Geometry check sheet. Reference: the model listing, model coordinates, mm. A direction names the side the tool comes from. Round coordinates to 2 decimals unless told otherwise and drop trailing zeros. Loops run counter-clockwise (first coordinate to the right, second up) from the corner with the lowest first, then second, coordinate; pieces in that order, holes last. Notation, with made-up numbers: (0, -33) - (59, -33) arc R25 ccw to (59, 2) - close; hole circle Ø10 at (-2, -14.5). An arc over 180 degrees is marked (long way). Write item = value, one per line.
```python
from build123d import *

# Parameters (mm, degrees)
SKETCH_W        = 22
SKETCH_H        = 30
PAD_DEPTH       = 27
SKETCH001_W     = 22
SKETCH001_H     = 28
PAD001_DEPTH    = 30
PAD002_DEPTH    = 4
SKETCH003_R     = 5
PAD003_DEPTH    = 4
PAD004_DEPTH    = 17
SKETCH005_R     = 7
PAD005_DEPTH    = 3
SKETCH006_R     = 4
POCKET_DEPTH    = 30
SKETCH007_W     = 15
SKETCH007_H     = 6
PAD006_DEPTH    = 5
SKETCH008_R     = 5
PAD007_DEPTH    = 4
PAD008_DEPTH    = 17
SKETCH010_R     = 7
PAD009_DEPTH    = 3
SKETCH011_R     = 4
POCKET001_DEPTH = 30
SKETCH012_R     = 2
POCKET002_DEPTH = 5


with BuildPart() as part:
    # Sketch → Pad (new body)
    with BuildSketch(Plane.XY):
        Rectangle(SKETCH_W, SKETCH_H)
    extrude(amount=PAD_DEPTH)

    # Sketch001 (on Face6 of Pad) → Pad001 (join)
    with BuildSketch(Plane.XY.offset(27)):
        with Locations((0, -1)):
            Rectangle(SKETCH001_W, SKETCH001_H)
    extrude(amount=PAD001_DEPTH)

    # Sketch002 (on Face11 of Pad001) → Pad002 (join)
    with BuildSketch(Plane.XY.offset(57)):
        Polygon((8.660254, -4), (4.330127, 3.5), (-4.330127, 3.5), (-8.660254, -4), (-4.330127, -11.5), (4.330127, -11.5), align=None)
    extrude(amount=PAD002_DEPTH)

    # Sketch003 (on Face6 of Pad002) → Pad003 (join)
    with BuildSketch(Plane.XZ.offset(15)):
        with Locations((0, 10)):
            Circle(SKETCH003_R)
    extrude(amount=PAD003_DEPTH)

    # Sketch004 (on Face13 of Pad003) → Pad004 (join)
    with BuildSketch(Plane.XZ.offset(19)):
        Polygon((8.082904, 10), (4.041452, 17), (-4.041452, 17), (-8.082904, 10), (-4.041452, 3), (4.041452, 3), align=None)
    extrude(amount=PAD004_DEPTH)

    # Sketch005 (on Face5 of Pad004) → Pad005 (join)
    with BuildSketch(Plane.XZ.offset(36)):
        with Locations((0, 10)):
            Circle(SKETCH005_R)
    extrude(amount=PAD005_DEPTH)

    # Sketch006 (on Face17 of Pad005) → Pocket (cut)
    with BuildSketch(Plane.XZ.offset(39)):
        with Locations((0, 10)):
            Circle(SKETCH006_R)
    extrude(amount=-POCKET_DEPTH, mode=Mode.SUBTRACT)

    # Sketch007 (on Face29 of Pocket) → Pad006 (join)
    with BuildSketch(Plane(origin=(0, 13, 0), x_dir=(-1, 0, 0), z_dir=(0, 1, 0))):
        with Locations((0, 50)):
            Rectangle(SKETCH007_W, SKETCH007_H)
    extrude(amount=PAD006_DEPTH)

    # Sketch008 (on Face23 of Pad006) → Pad007 (join)
    with BuildSketch(Plane(origin=(0, 15, 0), x_dir=(-1, 0, 0), z_dir=(0, 1, 0))):
        with Locations((0, 10)):
            Circle(SKETCH008_R)
    extrude(amount=PAD007_DEPTH)

    # Sketch009 (on Face37 of Pad007) → Pad008 (join)
    with BuildSketch(Plane(origin=(0, 19, 0), x_dir=(-1, 0, 0), z_dir=(0, 1, 0))):
        Polygon((4.041452, 3), (8.082904, 10), (4.041452, 17), (-4.041452, 17), (-8.082904, 10), (-4.041452, 3), align=None)
    extrude(amount=PAD008_DEPTH)

    # Sketch010 (on Face5 of Pad008) → Pad009 (join)
    with BuildSketch(Plane(origin=(0, 36, 0), x_dir=(-1, 0, 0), z_dir=(0, 1, 0))):
        with Locations((0, 10)):
            Circle(SKETCH010_R)
    extrude(amount=PAD009_DEPTH)

    # Sketch011 (on Face17 of Pad009) → Pocket001 (cut)
    with BuildSketch(Plane(origin=(0, 39, 0), x_dir=(-1, 0, 0), z_dir=(0, 1, 0))):
        with Locations((0, 10)):
            Circle(SKETCH011_R)
    extrude(amount=-POCKET001_DEPTH, mode=Mode.SUBTRACT)

    # Sketch012 (on Face19 of Pocket001) → Pocket002 (cut)
    with BuildSketch(Plane(origin=(0, 0, 0), x_dir=(1, 0, 0), z_dir=(0, 0, -1))):
        with Locations((-7.5, -11)):
            Circle(SKETCH012_R)
        with Locations((7.5, -11)):
            Circle(SKETCH012_R)
    extrude(amount=-POCKET002_DEPTH, mode=Mode.SUBTRACT)


solid = part.part
```
(1) Scan lines: L1, parallel to X at y = 11, z = 1; L2, parallel to Y at x = -7.5, z = 3.45; L3, parallel to Z at x = -0.25, y = 21.5. Record each from-to range of solid material in increasing order. Write a range as [from, to].
Answers follow:
L1 = [-11, -9.5], [-5.5, 5.5], [9.5, 11]
L2 = [-15, 9], [13, 15]
L3 = [3, 6.01], [13.99, 17]
(2) Mould release check, pull along X, two halves, no side actions. Record for faces 6 (the flat face through (-2, 19, 15)), 7 (the cylindrical face through (0.521, 24.21, 13.966)), 8 (the flat face through (-7.5, 15, 50)): pulls with the +X half, pulls with the -X half, needs draft (parallel to the pull), parting line crosses it, or undercut.
Answers follow:
face_6 = needs draft
face_7 = undercut
face_8 = pulls with the -X half
(3) Gauge pin test, flat ends, axial feed: pin 1 (4.5 mm diameter, centred on x = 7.5, y = 10, fed in from -Z); pin 2 (6.5 mm diameter, centred on x = 7.5, y = 11, fed in from +Z); pin 3 (1.2 mm diameter, centred on x = -7, y = 11.5, fed in from -Z); pin 4 (12 mm diameter, centred on x = 3, y = 27, fed in from -Z). Record the tip position at first contact, or that the pin passes through.
Answers follow:
pin_1 = 0
pin_2 = 57
pin_3 = 5
pin_4 = 3
(4) Section check B-B (z = 26). Enter the section's corners in (x, y), then the cut area to 3 significant figures.
Answers follow:
outline = (-11, -15) - (11, -15) - (11, 15) - (-11, 15) - close
area = 660 mm²
(5) Section check C-C (y = 34.5). Enter the section's corners in (x, z).
Answers follow:
outline = (-8.08, 10) - (-4.04, 3) - (4.04, 3) - (8.08, 10) - (4.04, 17) - (-4.04, 17) - close; hole circle Ø8 at (0, 10)
(6) Section check D-D (z = 56). Enter the section's corners in (x, y).
Answers follow:
outline = (-11, -15) - (11, -15) - (11, 13) - (-11, 13) - close
(7) Set-up check for faces 1 (the flat face through (0, 14, 27)), 2 (the flat face through (6.034, -27.381, 6.451)), 3 (the flat face through (-6.465, -0.198, 58.972)), 4 (the flat face through (-6.034, -27.381, 13.549)), 5 (the flat face through (3.5, 36, 16.3)): record each of +Z, -Z, +X, -X, +Y, -Y from which the full face is reachable in a straight line by a thin tool's end or side.
Answers follow:
face_1 = +X, -X, +Y
face_2 = -Z, +X, -Y
face_3 = +Z, -X, +Y
face_4 = +Z, -X, -Y
face_5 = +Z, +X, +Y
(8) Section check A-A (y = 11). Enter the section's corners in (x, z), then the cut area to 3 significant figures.
Answers follow:
outline = (-11, 0) - (-9.5, 0) - (-9.5, 5) - (-5.5, 5) - (-5.5, 0) - (5.5, 0) - (5.5, 5) - (9.5, 5) - (9.5, 0) - (11, 0) - (11, 57) - (-11, 57) - close; hole circle Ø8 at (0, 10)
area = 1,160 mm²
